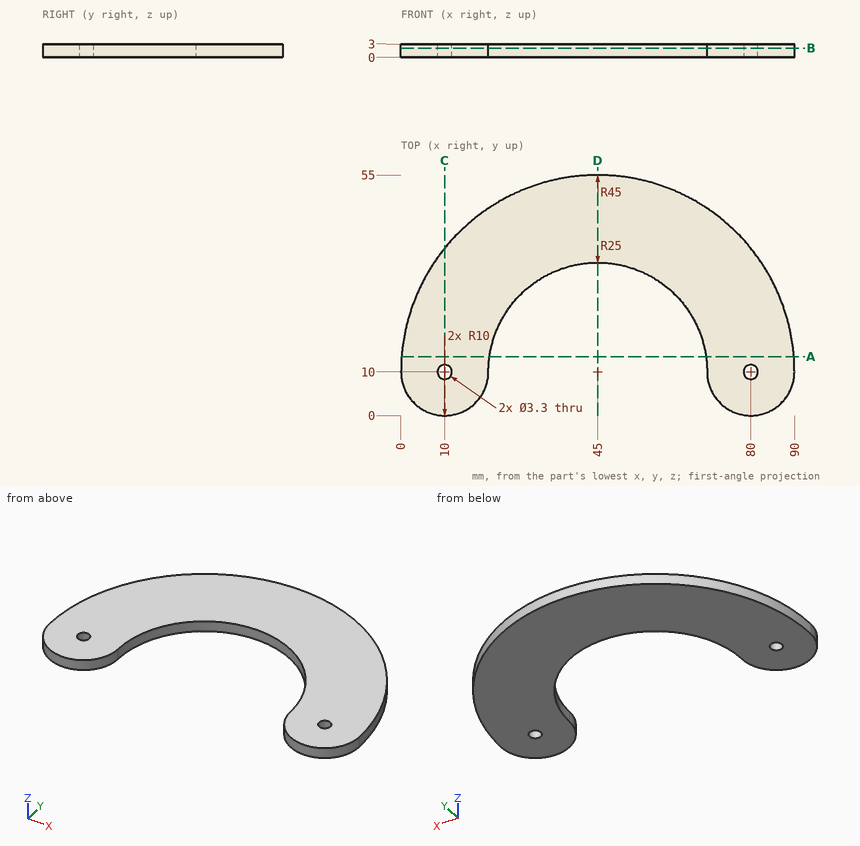
Can you work these out from the drawing? Everything is in mm from the part's minimum corner. Give positions to 0.01 mm unless a question says otherwise; leave off trailing zeros. Order: outer loops, then holes, each group sorted by start corner. A loop starts at its lowest first (then second) coordinate and runs counter-clockwise, first axis right, second up. Notation, with made-up numbers: (-27.5, 55) -> (-8.5, 55) arc R19 ccw to (-8.5, 84) -> close; hole circle Ø4 at (2.5, 52.25). An arc over 180 degrees is marked (long way). Return JSON: item names as keys, results as strings.
1. Imagine slicing it at C-C on x = 10. List the corners of the cut face in (y, z) for me.
Answer list:
{"outline": "(0, 0) -> (8.35, 0) -> (8.35, 3) -> (0, 3) -> close; (11.65, 0) -> (38.28, 0) -> (38.28, 3) -> (11.65, 3) -> close"}
2. Imagine slicing it at D-D on x = 45. List the corners of the cut face in (y, z) for me.
Answer list:
{"outline": "(35, 0) -> (55, 0) -> (55, 3) -> (35, 3) -> close"}
3. For pin 1 Ø6 at (x, y) = (66.5, 40) entering from -Z; pin 2 Ø10 at (x, y) = (38.5, 28.5) entering from -Z, each with a flat end and sliding along its axis, tell me the tip position at first contact or that it passes through.
Answer list:
{"pin 1": "stops at z = 0", "pin 2": "passes through"}
4. Imagine slicing it at A-A on y = 13.5. List the corners of the cut face in (x, z) for me.
Answer list:
{"outline": "(0.14, 0) -> (20.25, 0) -> (20.25, 3) -> (0.14, 3) -> close; (69.75, 0) -> (89.86, 0) -> (89.86, 3) -> (69.75, 3) -> close"}
5. I need wall thicknesses on line 1 (X direction, y = 30, z = 2.1); line 2 (X direction, y = 18.5, z = 1.75); line 3 (Y direction, x = 80, z = 2). Which ranges of each line are inside material? Lowest first, please. Write a range as from..to.
Answer list:
{"line 1": "x = 4.69..30, 60..85.31", "line 2": "x = 0.81..21.49, 68.51..89.19", "line 3": "y = 0..8.35, 11.65..38.28"}
6. Imagine slicing it at B-B on z = 2.05. List the corners of the cut face in (x, y) for me.
Answer list:
{"outline": "(0, 10) arc R10 ccw to (20, 10) arc R25 cw to (70, 10) arc R10 ccw to (90, 10) arc R45 ccw to start; hole circle Ø3.3 at (10, 10); hole circle Ø3.3 at (80, 10)"}
